Source: CAD feature listing. Evaluate the final solid. Frame: model axes, mm. A direction names the side the tool comes from. Give positions to 0.01 mm unless a question says otherwise; leave off trailing zeros. Write each loop counter-clockwise with the first axis right and the second up, starting at its lowest first coordinate (ties: lowest second). Pieces come first, ordered by that corner, then holes. Notation, with made-up numbers: (-8.5, 61.5) -> (18.5, 61.5) arc R22 ccw to (18.5, 82.5) -> close; hole circle Ø7 at (59, 80.5). An arc over 180 degrees is marked (long way). Answer as a JSON object with one key per item and string values. Group by question number.
Item 1: Access query for faces 1 (the face through (-0.027, -3.832, -1.777)), 2 (the face through (-2, -1, 0)), 3 (the face through (-1.78, -3.84, -0.03)). Directions: +Z, -Z, +X, -X, +Y, -Y. A direction counts if a zero-diameter tool reaches every point of the face in a straight line with its end or side. Return the directions, or none.
Item 2: Pull-direction query (Y, two-part tool) for faces 4 (the face through (4.94, 0.81, 1.3)), 5 (the face through (0, -5, 1.95)), 6 (the face through (1.777, -3.832, -0.027)); classes: pulls with the +Y half, pulls with the -Y half, needs draft (parallel to the pull), parting line crosses it, or undercut.
Item 3: Section query D-D on x = 6.75. Return the cut outline in (y, z), plus the area to 3 significant figures.
Item 4: Section query A-A on x = 0. Return the cut outline in (y, z), plus the area to 3 significant figures.
Item 5: Ray query, probe 1 along Z at (x, y) = (0.75, 0.75); probe 2 along Z at (x, y) = (-5, 0.75); probe 3 along X at (y, z) = (3.75, 0.05). Return the intervals inside material, ascending. Write a range as from..to.
Item 6: Section query C-C on y = 4.25. Return the cut outline in (x, z).
Item 7: First-contact query: pin 1 Ø1.5 at (x, z) = (3.5, 0) entering from -Y (3 decimals); pin 2 Ø0.9 at (x, y) = (1, -4.5) entering from +Z; pin 3 Ø1.5 at (x, z) = (4, 1) entering from +Y. Flat tips, straight axial feed; report the tip coordinate or a pass-through.
Item 8: Section query B-B on z = 0. Give the number of separate pieces and of enclosed holes in the cut face, plus the area to 3 significant figures.
from build123d import *

# Parameters (mm, degrees)
EXTRUDE_1_DEPTH          = 2
EXTRUDE_1_DEPTH_BACK     = 2
SKETCH_1_W               = 4
SKETCH_1_H               = 5.5
EXTRUDE_2_DEPTH          = 2
EXTRUDE_2_DEPTH_BACK     = 2
CUT_EXTRUDE_1_DEPTH      = 2
CUT_EXTRUDE_1_DEPTH_BACK = 2
SKETCH_4_R               = 1.4
SKETCH_5_R               = 1.2
SKETCH_6_R               = 1.4
SKETCH_7_R               = 1.2
SKETCH_8_R               = 0.8
CUT_EXTRUDE_2_DEPTH      = 19.345639944
SKETCH_9_R               = 0.8
CUT_EXTRUDE_3_DEPTH      = 8
FILLET_1_R               = 0.2
FILLET_2_R               = 0.2
FILLET_3_R               = 0.1


with BuildPart() as part:
    # 草图1 → 凸台-拉伸1 (new, two sides: drawn at the far end of the back side and taken through both)
    with BuildSketch(Plane.XY.offset(-EXTRUDE_1_DEPTH_BACK)):
        Rectangle(SKETCH_1_W, SKETCH_1_H)
    extrude(amount=EXTRUDE_1_DEPTH + EXTRUDE_1_DEPTH_BACK)

    # 草图2 → 凸台-拉伸2 (add, two sides: drawn at the far end of the back side and taken through both)
    with BuildSketch(Plane.XY.offset(-EXTRUDE_2_DEPTH_BACK)):
        with BuildLine():
            Line((-1.5, -2.75), (1.5, -2.75))
            Line((1.5, -2.75), (1.5, -3.427124344))
            ThreePointArc((1.5, -3.427124344), (1.780042303, -3.838161527), (1.95, -4.305590279))
            Line((1.95, -4.305590279), (1.95, -5.25))
            Line((1.95, -5.25), (-1.95, -5.25))
            Line((-1.95, -5.25), (-1.95, -4.305590279))
            ThreePointArc((-1.95, -4.305590279), (-1.780042303, -3.838161527), (-1.5, -3.427124344))
            Line((-1.5, -3.427124344), (-1.5, -2.75))
        make_face()
    extrude(amount=EXTRUDE_2_DEPTH + EXTRUDE_2_DEPTH_BACK)

    # 草图3 → 切除-拉伸1 (cut, two sides: drawn at the far end of the back side and taken through both)
    with BuildSketch(Plane(origin=(0, 0, 0), x_dir=(0, 0, -1), z_dir=(1, 0, 0)).offset(-CUT_EXTRUDE_1_DEPTH_BACK)):
        with BuildLine():
            Line((1.5, -2.75), (1.5, -3.427124344))
            ThreePointArc((1.5, -3.427124344), (1.780042303, -3.838161527), (1.95, -4.305590279))
            Line((1.95, -4.305590279), (1.95, -5.25))
            Line((1.95, -5.25), (2, -5.25))
            Line((2, -5.25), (2, -2.75))
            Line((2, -2.75), (1.5, -2.75))
        make_face()
        with BuildLine():
            Line((-2, -5.25), (-1.95, -5.25))
            Line((-1.95, -5.25), (-1.95, -4.305590279))
            ThreePointArc((-1.95, -4.305590279), (-1.780042303, -3.838161527), (-1.5, -3.427124344))
            Line((-1.5, -3.427124344), (-1.5, -2.75))
            Line((-1.5, -2.75), (-2, -2.75))
            Line((-2, -2.75), (-2, -5.25))
        make_face()
    extrude(amount=CUT_EXTRUDE_1_DEPTH + CUT_EXTRUDE_1_DEPTH_BACK, mode=Mode.SUBTRACT)

    # 草图4 → 放样2 section 0
    with BuildSketch(Plane(origin=(2, 0, 0), x_dir=(0, 0, -1), z_dir=(1, 0, 0))):
        with Locations((0, 0.75)):
            Circle(SKETCH_4_R)
    # 草图5 → 放样2 section 1
    with BuildSketch(Plane(origin=(8, 0, 0), x_dir=(0, 0, -1), z_dir=(1, 0, 0))):
        with Locations((0, 0.75)):
            Circle(SKETCH_5_R)
    loft_2 = loft()

    # 镜向1: 放样2 across plane
    add(loft_2.mirror(Plane(origin=(0, 0, 0), x_dir=(0, 0, 1), z_dir=(1, 0, 0))))

    # 草图6 → 放样3 section 0
    with BuildSketch(Plane(origin=(0, 2.75, 0), x_dir=(1, 0, 0), z_dir=(0, 1, 0))):
        Circle(SKETCH_6_R)
    # 草图7 → 放样3 section 1
    with BuildSketch(Plane(origin=(0, 8.75, 0), x_dir=(1, 0, 0), z_dir=(0, 1, 0))):
        Circle(SKETCH_7_R)
    loft()

    # 草图8 → 切除-拉伸2 (cut, through all)
    with BuildSketch(Plane(origin=(8, 0, 0), x_dir=(0, 0, -1), z_dir=(1, 0, 0))):
        with Locations(Location((0, 0.75, 0), (0, 0, 90))):
            Circle(SKETCH_8_R)
    extrude(amount=-CUT_EXTRUDE_2_DEPTH, mode=Mode.SUBTRACT)

    # 草图9 → 切除-拉伸3 (cut)
    with BuildSketch(Plane(origin=(0, 8.75, 0), x_dir=(1, 0, 0), z_dir=(0, 1, 0))):
        with Locations(Location((0, 0, 0), (0, 0, 270))):
            Circle(SKETCH_9_R)
    extrude(amount=-CUT_EXTRUDE_3_DEPTH, mode=Mode.SUBTRACT)

    # 圆角1
    fillet_1_edges = [part.edges().sort_by_distance(p)[0] for p in [
        (0, -2.75, -2),
        (0, 2.75, 2),
        (-2, 0, 2),
        (2, 0, -2),
        (0, -2.75, 2),
        (2, 0, 2),
        (0, 2.75, -2),
        (-2, 0, -2),
        (2, 2.75, 0),
        (2, -2.75, 0),
        (-2, -2.75, 0),
        (-2, 2.75, 0),
    ]]
    fillet(fillet_1_edges, radius=FILLET_1_R)

    # 圆角2
    fillet_2_edges = [part.edges().sort_by_distance(p)[0] for p in [
        (8, 0.75, 1.2),
        (-8, 0.75, 1.2),
        (-1.2, 8.75, 0),
    ]]
    fillet(fillet_2_edges, radius=FILLET_2_R)

    # 圆角3
    fillet_3_edges = [part.edges().sort_by_distance(p)[0] for p in [
        (0, -5.25, 1.95),
        (1.95, -5.25, 0),
        (-1.95, -5.25, 0),
        (0, -5.25, -1.95),
    ]]
    fillet(fillet_3_edges, radius=FILLET_3_R)


solid = part.part
Worked answers:
{
 "1": {"face 1": "-Z, +X, -X", "face 2": "-X", "face 3": "+Z, -Z, -X"},
 "2": {"face 4": "parting line crosses it", "face 5": "needs draft", "face 6": "undercut"},
 "3": {"outline": "circle Ø2.48 at (0.75, 0); hole circle Ø1.6 at (0.75, 0)", "area": "2.83 mm^2"},
 "4": {"outline": "(-5.25, -1.85) arc R0.1 ccw to (-5.15, -1.95) -> (-4.31, -1.95) arc R2 ccw to (-3.43, -1.5) -> (-2.75, -1.5) -> (-2.75, -1.8) arc R0.2 ccw to (-2.55, -2) -> (2.55, -2) arc R0.2 ccw to (2.75, -1.8) -> (2.75, -1.4) -> (8.56, -1.21) arc R0.2 ccw to (8.75, -1.01) -> (8.75, -0.8) -> (0.75, -0.8) arc R0.8 cw to (0.75, 0.8) -> (8.75, 0.8) -> (8.75, 1.01) arc R0.2 ccw to (8.56, 1.21) -> (2.75, 1.4) -> (2.75, 1.8) arc R0.2 ccw to (2.55, 2) -> (-2.55, 2) arc R0.2 ccw to (-2.75, 1.8) -> (-2.75, 1.5) -> (-3.43, 1.5) arc R2 ccw to (-4.31, 1.95) -> (-5.15, 1.95) arc R0.1 ccw to (-5.25, 1.85) -> close", "area": "32.6 mm^2"},
 "5": {"probe 1": "-2..-0.8, 0.8..2", "probe 2": "-1.3..-0.8, 0.8..1.3", "probe 3": "-1.37..-0.8, 0.8..1.37"},
 "6": {"outline": "circle Ø2.7 at (0, 0); hole circle Ø1.6 at (0, 0)"},
 "7": {"pin 1": "y = -0.625", "pin 2": "z = 1.95", "pin 3": "y = 2.06"},
 "8": {"separate pieces": "3", "enclosed holes": "0", "area": "40.4 mm^2"}
}
